Autodesk Inventor part; units mm, degrees
ref_plane "YZ Plane" through (0, 0, 0) normal (1, 0, 0) x (0, 1, 0)
ref_plane "XZ Plane" through (0, 0, 0) normal (0, 1, 0) x (-1, 0, 0)
ref_plane "XY Plane" through (0, 0, 0) normal (0, 0, 1) x (1, 0, 0)
sketch "Sketch14" plane through (0, 0, 0) normal (0, 0, 1) x (1, 0, 0)
  line L0 (0, 0) -> (-6.08, 0)
  line L1 (-6.08, 0) -> (0, 0)
  line L2 (0, 0) -> (6.08, 0)
  line L3 (-6.08, 0) -> (-6.08, 5)
  line L4 (-6.08, 0) -> (-1.08, 0) construction
  line L5 (-6.08, 5) -> (6.08, 5)
  line L6 (6.08, 5) -> (6.08, -5)
  line L7 (6.08, -5) -> (-6.08, -5)
  line L8 (-6.08, -5) -> (-6.08, 5)
  dimension "d66" = 6.08
  dimension "d67" = 6.08
  dimension "d68" = 5
  dimension "d69" = 90
  dimension "d70" = 12.16
  dimension "d71" = 10
extrude "Extrusion7" add sketch "Sketch14" along normal blind 2
sketch "Sketch15" plane through (0, 0, 2) normal (0, 0, 1) x (1, 0, 0)
  circle A0 centre (0, 0) radius 1.0665
hole "Hole4" at (0, 0, 2) direction (0, 0, -1) diameter 4.5 end through all
sketch "Sketch16" plane through (0, 0, 2) normal (0, 0, 1) x (1, 0, 0)
  line L0 (6.08, 5) -> (-6.08, 5)
  line L1 (0, 5) -> (10, 5)
  line L2 (10, 5) -> (-25.7, 5)
  line L3 (-25.7, 5) -> (-25.7, 37.05)
  line L4 (-25.7, 37.05) -> (10, 37.05)
  line L5 (10, 37.05) -> (10, 5)
  line L6 (-6.08, -5) -> (6.08, -5)
  line L7 (0, -5) -> (10, -5)
  line L8 (10, -5) -> (-25.7, -5)
  line L9 (-25.7, -5) -> (-25.7, -37.05)
  line L10 (-25.7, -37.05) -> (10, -37.05)
  line L11 (10, -37.05) -> (10, -5)
  line L12 (-25.7, 37.05) -> (-22.7, 37.05)
  line L13 (-22.7, 37.05) -> (-22.7, 34.05)
  line L14 (-22.7, 34.05) -> (-25.7, 34.05)
  line L15 (-25.7, 34.05) -> (-25.7, 37.05)
  line L16 (-22.7, 34.05) -> (7, 34.05)
  line L17 (7, 34.05) -> (7, 8)
  line L18 (7, 8) -> (-22.7, 8)
  line L19 (-22.7, 8) -> (-22.7, 34.05)
  line L20 (-25.7, -37.05) -> (-22.7, -37.05)
  line L21 (-22.7, -37.05) -> (-22.7, -34.05)
  line L22 (-22.7, -34.05) -> (-25.7, -34.05)
  line L23 (-25.7, -34.05) -> (-25.7, -37.05)
  line L24 (-22.7, -34.05) -> (7, -34.05)
  line L25 (7, -34.05) -> (7, -8)
  line L26 (7, -8) -> (-22.7, -8)
  line L27 (-22.7, -8) -> (-22.7, -34.05)
  line L28 (-25.7, -5) -> (10, -5)
  line L29 (10, -5) -> (10, -37.05)
  line L30 (10, -37.05) -> (-25.7, -37.05)
  line L31 (-25.7, -37.05) -> (-25.7, -5)
  point P0 (0, 0)
  dimension "d81" = 10
  dimension "d82" = 35.7
  dimension "d83" = 32.05
  dimension "d84" = 35.7
  dimension "d85" = 32.05
  dimension "d86" = 3
  dimension "d87" = 3
  dimension "d88" = 29.7
  dimension "d89" = 26.05
  dimension "d90" = 3
  dimension "d91" = 3
  dimension "d92" = 29.7
  dimension "d93" = 26.05
  dimension "d172" = 10
extrude "Extrusion8" add sketch "Sketch16" along normal blind 1.5 contours L16 L17 L18 L19 | L0 L2 L3 L14 L13 L4 L5 L1 | L13 L14 L3 L4 | L27 L26 L25 L24 | L6 L7 L11 L10 L21 L22 L9 L8 | L22 L21 L10 L9
hole "Hole5" at (-22.7, 34.05, 2) at (-22.7, 8, 2) at (7, 8, 2) at (7, 34.05, 2) at (7, -8, 2) at (7, -34.05, 2) at (-22.7, -34.05, 2) at (-22.7, -8, 2) direction (0, 0, 1) diameter 3.9 end through all
sketch "Sketch17" plane through (0, 0, 2) normal (0, 0, 1) x (1, 0, 0)
  circle A0 centre (0, 0) radius 2.25
  line L0 (6.08, -5) -> (6.08, 5)
  line L1 (6.08, 5) -> (-6.08, 5)
  line L2 (-6.08, 5) -> (-6.08, -5)
  line L3 (-6.08, -5) -> (6.08, -5)
extrude "Extrusion9" add sketch "Sketch17" along normal blind 4
sketch "Sketch18" plane through (6.08, -5, 0) normal (1, 0, 0) x (0, 0, -1)
  line L0 (0, 0) -> (0, 10)
  line L1 (0, 10) -> (-2, 10)
  line L2 (-3.5, 10) -> (-2, 10)
  line L3 (-3.5, 10) -> (-6, 10)
  line L4 (-6, 0) -> (-6, 10)
  line L5 (-3.5, 0) -> (-6, 0)
  line L6 (-2, 0) -> (-3.5, 0)
  line L7 (0, 0) -> (-2, 0)
  point P0 (0, 5)
extrude "Extrusion10" add sketch "Sketch18" along normal blind 35
sketch "Sketch19" plane through (41.08, -5, 0) normal (1, 0, 0) x (0, 0, -1)
  line L0 (-6, 10) -> (-6, 0)
  line L1 (-6, 0) -> (-16, 0)
  line L2 (-16, 0) -> (-16, 50)
  line L3 (-16, 50) -> (29, 50)
  line L4 (29, 50) -> (29, 25)
  line L5 (29, 25) -> (0, 10)
  line L6 (0, 10) -> (0, 0)
  line L7 (0, 10) -> (0, 0)
  line L8 (0, 0) -> (-6, 0)
  point P0 (0, 5)
  dimension "d107" = 10
  dimension "d108" = 50
  dimension "d109" = 90
  dimension "d110" = 45
  dimension "d111" = 90
  dimension "d112" = 25
extrude "Extrusion11" add sketch "Sketch19" along normal blind 2.5
sketch "Sketch21" plane through (43.58, -5, 0) normal (1, 0, 0) x (0, 0, -1)
  line L0 (-3.5, 10) -> (-6, 10)
  line L1 (0, 10) -> (0, 24.05)
  line L2 (0, 10) -> (14.05, 10) construction
  line L3 (0, 24.05) -> (6.713, 24.05)
  point P0 (0, 5)
  point P1 (3, 10)
  point P2 (-2, 10)
  dimension "d118" = 14.05
  dimension "d119" = 90
  dimension "d120" = 6.713
  dimension "d121" = 90
hole "Hole6" at (43.58, 19.05, -6.713) direction (-1, 0, 0) diameter 10 end through all
sketch "Sketch22" plane through (43.58, -5, 0) normal (1, 0, 0) x (0, 0, -1)
  circle A0 centre (6.713, 24.05) radius 5
  line L0 (6.713, 24.05) -> (6.713, 32.05)
  line L1 (6.713, 24.05) -> (14.713, 24.05) construction
  line L2 (6.713, 32.05) -> (24.213, 32.05)
  line L3 (24.213, 32.05) -> (-10.787, 32.05)
  point P0 (0, 5)
  dimension "d129" = 8
  dimension "d130" = 90
  dimension "d131" = 17.5
  dimension "d132" = 90
  dimension "d133" = 35
hole "Hole7" at (43.58, 27.05, 10.787) at (43.58, 27.05, -24.213) direction (-1, 0, 0) diameter 4.2 end through all
sketch "Sketch23" plane through (43.58, -5, 0) normal (1, 0, 0) x (0, 0, -1)
  line L0 (-3.5, 0) -> (-2, 0)
  line L1 (-2, 0) -> (-2, -9)
  line L2 (-2, 0) -> (7, 0) construction
  line L3 (-2, -9) -> (33, -9) construction
  line L4 (-2, -9) -> (33, -9)
  line L5 (-2, -9) -> (33, -9) construction
  line L6 (33, -9) -> (40.7782, -1.2218)
  line L7 (40.7782, -1.2218) -> (60.7782, -1.2218)
  line L8 (33, -9) -> (68, -9)
  line L9 (33, -9) -> (68, -9) construction
  line L10 (68, -9) -> (68, -1.2218)
  line L11 (68, -1.2218) -> (60.7782, -1.2218)
  line L12 (68, -9) -> (68, -29)
  line L13 (68, -9) -> (88, -9) construction
  line L14 (68, -29) -> (-2, -29)
  line L15 (-2, -29) -> (-2, -9)
  line L16 (33, -9) -> (44.45, -9)
  line L17 (44.45, -9) -> (44.45, -13.669)
  line L18 (44.45, -9) -> (49.119, -9) construction
  line L19 (44.45, -13.669) -> (44.45, -21.669)
  line L20 (44.45, -21.669) -> (61.95, -21.669)
  line L21 (61.95, -21.669) -> (26.95, -21.669)
  circle A0 centre (26.95, -21.669) radius 2.1
  circle A1 centre (61.95, -21.669) radius 2.1
  circle A2 centre (44.45, -13.669) radius 5
  point P0 (0, 5)
  dimension "d141" = 9
  dimension "d142" = 90
  dimension "d145" = 35
  dimension "d146" = 0
  dimension "d147" = 11
  dimension "d148" = 135
  dimension "d149" = 20
  dimension "d150" = 35
  dimension "d151" = 0
  dimension "d152" = 20
  dimension "d153" = 90
  dimension "d154" = 90
  dimension "d155" = 11.45
  dimension "d156" = 4.669
  dimension "d157" = 90
  dimension "d158" = 8
  dimension "d159" = 17.5
  dimension "d160" = 35
  dimension "d161" = 4.2
  dimension "d162" = 4.2
  dimension "d163" = 10
extrude "Extrusion13" add sketch "Sketch23" against normal blind 2 contours L4 L8 A2 L12 L14 L15 | L6 L7 L11 L10 L8 A2
sketch "Sketch24" plane through (43.58, -5, 0) normal (1, 0, 0) x (0, 0, -1)
  line L0 (-16, 50) -> (-16, 0)
  line L1 (-16, 0) -> (-16, -29)
  line L2 (68, -29) -> (-2, -29)
  line L3 (-16, -29) -> (-2, -29)
  line L4 (0, 0) -> (-2, 0)
  line L5 (-2, -29) -> (-2, 0)
  line L6 (-16, 0) -> (0, 0)
  line L7 (-2, 0) -> (-16, 0)
  point P0 (0, 5)
  point P1 (3, 0)
extrude "Extrusion14" add sketch "Sketch24" against normal blind 2
sketch "Sketch25" plane through (41.58, -5, 0) normal (-1, 0, 0) x (0, 0, 1)
  line L0 (2, -9) -> (-33, -9)
  line L1 (-33, -9) -> (2, -9)
  line L2 (2, -9) -> (2, -11)
  line L3 (2, -11) -> (-33, -11)
  line L4 (-33, -11) -> (-33, -9)
  line L5 (2, -11) -> (6, -11)
  line L6 (6, -11) -> (6, 0)
  line L7 (6, 0) -> (2, 0)
  line L8 (2, 0) -> (2, -11)
  point P0 (0, 5)
  point P1 (2, -9)
  dimension "d168" = 35
  dimension "d169" = 2
extrude "Extrusion15" add sketch "Sketch25" along normal blind 10
properties part number "Shelf"
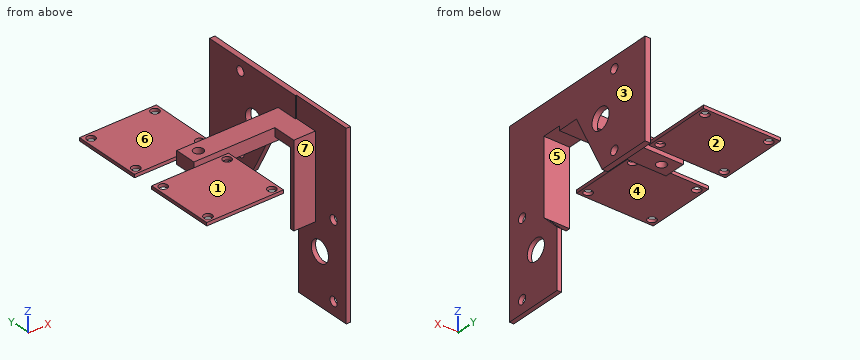
CAD build for the part. Positions are in the model's coordinates, mm. Face numbers are marked on the shaded views. A direction names the side the tool comes from. Round coordinates to 2 decimals unless told otherwise and drop trailing zeros. Order: outer loops, then holes, each group sorted by start corner. A loop starts at its lowest first (then second) coordinate and runs counter-clockwise, first axis right, second up.
Item 1: Saw through at B-B on z = -44.45. Write the cut outline in (x, y), then the cut area to 3 significant figures.
Item 2: Mould opens along Y. For the marked faces 5, 6 and 7 say: pulls with the +Y half, pulls with the -Y half, needs draft (parallel to the pull), parting line crosses it, or undercut.
Item 3: Probe line 1 along Y through (x, z) = (-22.7, 2.8); line 2 along Z through (x, y) = (42, 27); line 3 along Y through (x, z) = (42, -44). List the from-to ranges inside material, lowest first.
Item 4: Saw through at C-C on x = -14. Write the cut outline in (y, z).
Item 5: Saw through at D-D on x = 7. Write the cut outline in (y, z), then the cut area to 3 significant figures.
Item 6: Saw through at A-A on y = 0. Write the cut outline in (x, z), then the cut area to 3 significant figures.
Item 7: Pin check, flat tips, straight feed: pin 1 (2 mm diameter, centred on x = 37.5, y = -14.5, fed in from -Z); pin 2 (5 mm diameter, centred on x = 21, z = 3, fed in from +Y); pin 3 (5 mm diameter, centred on x = 7, y = -34.05, fed in from -Z). Stop position of each tip, or through.
Item 8: Tool access for the marked faces 1, 2, 3 and 4: list every direction of +Z, -Z, +X, -X, +Y, -Y with a clear straight run to the whole face (end or side of a thin tool).
Reported:
1. outline: (41.58, -34) - (43.58, -34) - (43.58, -23.67) - (41.58, -23.67) - close; (41.58, -13.67) - (43.58, -13.67) - (43.58, -6.22) - (41.58, -6.22) - close
1. area: 35.6 mm2
2. face 5: undercut
2. face 6: needs draft
2. face 7: pulls with the -Y half
3. line 1: y = -37.05 to -36, -32.1 to -9.95, -6.05 to -5, 5 to 6.05, 9.95 to 32.1, 36 to 37.05
3. line 2: z = -29 to -26.31, -22.11 to 8.69, 12.89 to 16
3. line 3: y = -34 to -23.65, -13.69 to -6.22
4. outline: (-37.05, 2) - (-5, 2) - (-5, 3.5) - (-37.05, 3.5) - close; (5, 2) - (37.05, 2) - (37.05, 3.5) - (5, 3.5) - close
5. outline: (-37.05, 2) - (-36, 2) - (-36, 3.5) - (-37.05, 3.5) - close; (-32.1, 2) - (-9.95, 2) - (-9.95, 3.5) - (-32.1, 3.5) - close; (-6.05, 2) - (-5, 2) - (-5, 0) - (5, 0) - (5, 2) - (6.05, 2) - (6.05, 3.5) - (5, 3.5) - (5, 6) - (-5, 6) - (-5, 3.5) - (-6.05, 3.5) - close; (9.95, 2) - (32.1, 2) - (32.1, 3.5) - (9.95, 3.5) - close; (36, 2) - (37.05, 2) - (37.05, 3.5) - (36, 3.5) - close
5. area: 133 mm2
6. outline: (-6.08, 0) - (-2.25, 0) - (-2.25, 6) - (-6.08, 6) - close; (2.25, 0) - (43.58, 0) - (43.58, 16) - (41.08, 16) - (41.08, 6) - (2.25, 6) - close
6. area: 296 mm2
7. pin 1: stops at z = -33
7. pin 2: stops at y = 5
7. pin 3: stops at z = 2
8. face 1: +Z, -X, -Y
8. face 2: -Z, -X, +Y
8. face 3: +Z, -Z, +X, +Y, -Y
8. face 4: -Z, -X, -Y
